Part model, mm, in its own coordinate system. Give positions to 0.01 mm unless a question says otherwise; leave off trailing zeros. Loops run counter-clockwise (first coordinate to the right, second up) from the corner with the lowest first, then second, coordinate; pieces in that order, holes last. Notation, with made-up numbers: M 39.25,1 L 90.25,1 A30 cw 90.25,35 Z; hole C 42.5,42 d6. An arc over 180 degrees is marked long. Put each result on its own line as item: value. Start each with the question number.
```python
from build123d import *

# Parameters (mm, degrees)
SKETCH1_W       = 305
SKETCH1_H       = 945
EXTRUDE1_DEPTH  = 3
SKETCH2_R       = 114.37
SKETCH2_R_2     = 110.37
EXTRUDE2_DEPTH  = 15
SKETCH3_W       = 3
SKETCH3_H       = 15
EXTRUDE3_DEPTH  = 125
SKETCH4_W       = 3
SKETCH4_H       = 5
SKETCH4_H_2     = 6
SKETCH4_W_2     = 74.4375
SKETCH4_H_3     = 3.826546867
SKETCH4_H_4     = 3.798552334
SKETCH4_W_3     = 55.3875
SKETCH4_H_5     = 4.7625
SKETCH4_H_6     = 3.8875
EXTRUDE4_DEPTH  = 4
SKETCH5_W       = 3
SKETCH5_H       = 170
EXTRUDE5_DEPTH  = 203
SKETCH6_W       = 3
SKETCH6_H       = 170
EXTRUDE6_DEPTH  = 30
EXTRUDE7_DEPTH  = 19
SKETCH13_R      = 88.098729295
EXTRUDE10_DEPTH = 207
SKETCH22_R      = 116.4
SKETCH22_R_2    = 112.37
EXTRUDE17_DEPTH = 5
SKETCH23_R      = 114.37
SKETCH23_R_2    = 110.37
EXTRUDE18_DEPTH = 15


with BuildPart() as part:
    # Sketch1 → Extrude1 (new body)
    with BuildSketch(Plane.XY):
        with Locations((152.5, 472.5)):
            Rectangle(SKETCH1_W, SKETCH1_H)
    extrude(amount=EXTRUDE1_DEPTH)

    # Sketch2 → Extrude2 (add)
    with BuildSketch(Plane.XY.offset(3)):
        with Locations((78, 472.5)):
            Circle(SKETCH2_R)
        with Locations((78, 472.5)):
            Circle(SKETCH2_R_2, mode=Mode.SUBTRACT)
    extrude(amount=EXTRUDE2_DEPTH)

    # Sketch3 → Extrude3 (add)
    with BuildSketch(Plane(origin=(0, 0, 0), x_dir=(-1, 0, 0), z_dir=(0, 0, -1))):
        with Locations((-2.5, 937.5)):
            Rectangle(SKETCH3_W, SKETCH3_H)
        with Locations((-2.5, 7.5)):
            Rectangle(SKETCH3_W, SKETCH3_H)
    extrude(amount=EXTRUDE3_DEPTH)

    # Sketch4 → Extrude4 (add)
    with BuildSketch(Plane(origin=(4, 0, 0), x_dir=(0, 0, -1), z_dir=(1, 0, 0))):
        with Locations((123.5, 942.5)):
            Rectangle(SKETCH4_W, SKETCH4_H)
        with Locations((123.5, 3)):
            Rectangle(SKETCH4_W, SKETCH4_H_2)
        with Locations((34.21875, 943.086726567)):
            Rectangle(SKETCH4_W_2, SKETCH4_H_3)
        with Locations((34.21875, 931.899276167)):
            Rectangle(SKETCH4_W_2, SKETCH4_H_4)
        with Locations((24.69375, 2.38125)):
            Rectangle(SKETCH4_W_3, SKETCH4_H_5)
        with Locations((24.69375, 13.05625)):
            Rectangle(SKETCH4_W_3, SKETCH4_H_6)
    extrude(amount=EXTRUDE4_DEPTH)

    # Sketch5 → Extrude5 (add)
    with BuildSketch(Plane(origin=(0, 0, 0), x_dir=(-1, 0, 0), z_dir=(0, 0, -1))):
        with Locations((-303.5, 472.5)):
            Rectangle(SKETCH5_W, SKETCH5_H)
    extrude(amount=EXTRUDE5_DEPTH)

    # Sketch6 → Extrude6 (add)
    with BuildSketch(Plane.ZY.offset(-302)):
        with Locations((-201.5, 472.5)):
            Rectangle(SKETCH6_W, SKETCH6_H)
    extrude(amount=EXTRUDE6_DEPTH)

    # Sketch7 → Extrude7 (cut, through all)
    with BuildSketch(Plane(origin=(0, 0, 0), x_dir=(-1, 0, 0), z_dir=(0, 0, -1))):
        Polygon((-305, 557.5), (-63.714944106, 945), (-305, 945), align=None)
        Polygon((-305, 387.5), (-63.714944106, 0), (-305, 0), align=None)
    extrude(amount=-EXTRUDE7_DEPTH, mode=Mode.SUBTRACT)

    # Sketch13 → Extrude10 (cut, through all)
    with BuildSketch(Plane.XY.offset(3)):
        with Locations((78, 472.5)):
            Circle(SKETCH13_R)
    extrude(amount=-EXTRUDE10_DEPTH, mode=Mode.SUBTRACT)

    # Sketch22 → Extrude17 (add)
    with BuildSketch(Plane.XY.offset(18)):
        with Locations((78, 472.5)):
            Circle(SKETCH22_R)
        with Locations((78, 472.5)):
            Circle(SKETCH22_R_2, mode=Mode.SUBTRACT)
    extrude(amount=EXTRUDE17_DEPTH)

    # Sketch23 → Extrude18 (add)
    with BuildSketch(Plane.XY.offset(23)):
        with Locations((78, 472.5)):
            Circle(SKETCH23_R)
        with Locations((78, 472.5)):
            Circle(SKETCH23_R_2, mode=Mode.SUBTRACT)
    extrude(amount=EXTRUDE18_DEPTH)


solid = part.part
```
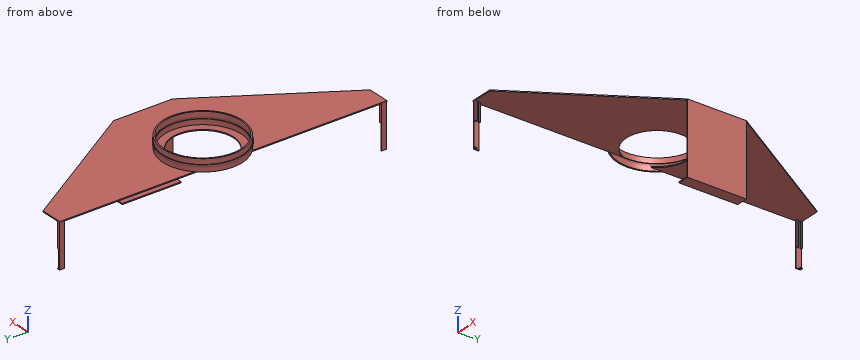
1) Band-saw the part on D-D on z = -180.5. Give the cut face in (x, y), then the cut area to 3 significant figures.
2) Band-saw the part on A-A on z = -85.5. Give the cut face in (x, y).
3) Pin check, flat tips, straight feed: pin 1 Ø7.5 at (x, y) = (5, 4.5) entering from -Z; pin 2 Ø16.5 at (x, z) = (295, -52) entering from +Y; pin 3 Ø3 at (x, y) = (180, 519) entering from -Z; pin 4 Ø1.5 at (x, z) = (5.5, -123.5) entering from -Y. Stop position of each tip, or through.
4) Wall check: L1, parallel to Y at x = 78, z = 32; L2, parallel to Y at x = 78, z = 20.2; L3, parallel to Z at x = 33, y = 591. Give the ranges that are in metal, low to high.
Evaluation:
1. outline: M 302,387.5 L 305,387.5 L 305,557.5 L 302,557.5 Z
1. area: 510 mm2
2. outline: M 1,0 L 4,0 L 4,15 L 1,15 Z; M 1,930 L 4,930 L 4,945 L 1,945 Z; M 302,387.5 L 305,387.5 L 305,557.5 L 302,557.5 Z
3. pin 1: z = -125
3. pin 2: y = 557.5
3. pin 3: z = 0
3. pin 4: y = 0
4. L1: 358.13 to 362.13, 582.87 to 586.87
4. L2: 356.1 to 360.13, 584.87 to 588.9
4. L3: 0 to 3
